Here's how the part is built. I have some questions about the finished solid (model axes, mm). Face numbers are marked on the shaded views. A direction names the side the tool comes from. Coordinates: 2 decimals unless noted, no trailing zeros. Loops run counter-clockwise (first coordinate to the right, second up) from the corner with the lowest first, then second, coordinate; pieces in that order, holes last. Notation, with made-up numbers: M 13,-29 L 34,-29 A28 cw 34,-11 Z; hole C 0,9 d9. An arc over 180 degrees is marked long. Use CSV: the item, a comma, the result in double quotes. Start each with the question number.
Q1. If we section it at A-A (z = -11): Please give me the cut outline in (x, y), and give its area (3 significant figures).
Q2. If we mould it in two halves opening along X, with no side actions, what happens to the marked faces 1, 2, 3 and 4? For each: +X half, -X half, draft (parallel to the pull), parting line (faces both ways), or undercut.
Q3. If we section it at B-B (x = 0): Please give me the cut outline in (y, z).
Q4. If we section it at C-C (z = 0): Please give me the cut outline in (x, y).
Q5. If we section it at D-D (y = 62.5): State how many separate pieces and enclosed holes the cut face has, and give its area (3 significant figures).
Q6. Which directions (+Z, -Z, +X, -X, +Y, -Y) give clear straight access to the entire face, cutting with the end or side of a thin tool? Please do the marked faces 5 and 6.
Q7. For pin 1 Ø6 at (y, z) = (30, 1) entering from +X; pin 2 Ø2.5 at (y, z) = (24, -0.5) entering from -X, each with a flat end and sliding along its axis, tell me the tip position at first contact or that it passes through.
Q8. Please list where these lines run through material, in increasing order: probe 1 along X at (y, z) = (39, 0); probe 2 along Z at (x, y) = (-11, 8.5). Write a range as [from, to].
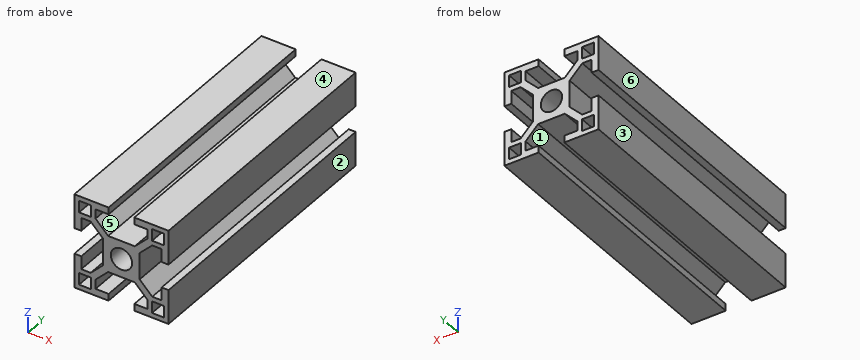
from build123d import *

# Parameters (mm, degrees)
SZKIC1_R                    = 3.4
SZKIC1_W                    = 3.75
SZKIC1_H                    = 3.75
DODANIE_WYCI_GNI_CIE1_DEPTH = 88


with BuildPart() as part:
    # Szkic1 → Dodanie-wyciągnięcie1 (new body)
    with BuildSketch(Plane(origin=(0, 0, 0), x_dir=(1, 0, 0), z_dir=(0, 1, 0))):
        Polygon((4.1, 15), (4.1, 12.8), (8.25, 12.8), (8.25, 9.805634919), (4.244365081, 5.8), (-4.244365081, 5.8), (-8.25, 9.805634919), (-8.25, 12.8), (-4.1, 12.8), (-4.1, 15), (-15, 15), (-15, 4.1), (-12.8, 4.1), (-12.8, 8.25), (-9.805634919, 8.25), (-5.8, 4.244365081), (-5.8, -4.244365081), (-9.805634919, -8.25), (-12.8, -8.25), (-12.8, -4.1), (-15, -4.1), (-15, -15), (-4.1, -15), (-4.1, -12.8), (-8.25, -12.8), (-8.25, -9.805634919), (-4.244365081, -5.8), (4.244365081, -5.8), (8.25, -9.805634919), (8.25, -12.8), (4.1, -12.8), (4.1, -15), (15, -15), (15, -4.1), (12.8, -4.1), (12.8, -8.25), (9.805634919, -8.25), (5.8, -4.244365081), (5.8, 4.244365081), (9.805634919, 8.25), (12.8, 8.25), (12.8, 4.1), (15, 4.1), (15, 15), align=None)
        Circle(SZKIC1_R, mode=Mode.SUBTRACT)
        with Locations((11.625, 11.625)):
            Rectangle(SZKIC1_W, SZKIC1_H, mode=Mode.SUBTRACT)
        with Locations((11.625, -11.625)):
            Rectangle(SZKIC1_W, SZKIC1_H, mode=Mode.SUBTRACT)
        with Locations((-11.625, -11.625)):
            Rectangle(SZKIC1_W, SZKIC1_H, mode=Mode.SUBTRACT)
        with Locations((-11.625, 11.625)):
            Rectangle(SZKIC1_W, SZKIC1_H, mode=Mode.SUBTRACT)
    extrude(amount=DODANIE_WYCI_GNI_CIE1_DEPTH)


solid = part.part
Results below:
1,outline,"M -15,0 L -13.5,0 L -13.5,88 L -15,88 Z; M -9.75,0 L -8.25,0 L -8.25,88 L -9.75,88 Z; M 8.25,0 L 9.75,0 L 9.75,88 L 8.25,88 Z; M 13.5,0 L 15,0 L 15,88 L 13.5,88 Z"
1,area,"528 mm^2"
2,face 1,"undercut"
2,face 2,"+X half"
2,face 3,"-X half"
2,face 4,"draft"
3,outline,"M 0,-5.8 L 88,-5.8 L 88,-3.4 L 0,-3.4 Z; M 0,3.4 L 88,3.4 L 88,5.8 L 0,5.8 Z"
4,outline,"M -5.8,0 L -3.4,0 L -3.4,88 L -5.8,88 Z; M 3.4,0 L 5.8,0 L 5.8,88 L 3.4,88 Z"
5,separate pieces,"1"
5,enclosed holes,"5"
5,area,"337 mm^2"
6,face 5,"+Y, -Y"
6,face 6,"+Z, -Z, -X, +Y, -Y"
7,pin 1,"x = 5.8"
7,pin 2,"x = -5.8"
8,probe 1,"[-5.8, -3.4], [3.4, 5.8]"
8,probe 2,"[-15, -13.5], [-9.75, -8.25], [8.25, 9.75], [13.5, 15]"
